```python
from build123d import *

# Parameters (mm, degrees)
F1_DEPTH = 30
F2_R     = 10
F3_R     = 10
F4_R     = 10
F5_R     = 10
F6_W     = 10
F6_H     = 10
F6_R     = 0.75
F7_DEPTH = 2


with BuildPart() as f1:
    # F0 (on Front) → F1 (new body)
    with BuildSketch(Plane.XZ):
        Polygon((40, 0), (0, 0), (-40, 0), (-48.660254, 5), (-51.324189, 0.768753), (-41.332416, -5), (41.336155, -5), (51.275389, 0.73842), (48.660254, 5), align=None)
    extrude(amount=F1_DEPTH)

    # F2
    f2_edges = [f1.edges().sort_by_distance(p)[0] for p in [
        (49.967822, -30, 2.86921),
    ]]
    fillet(f2_edges, radius=F2_R)

    # F3
    f3_edges = [f1.edges().sort_by_distance(p)[0] for p in [
        (49.967822, 0, 2.86921),
    ]]
    fillet(f3_edges, radius=F3_R)

    # F4
    f4_edges = [f1.edges().sort_by_distance(p)[0] for p in [
        (-49.992221, 0, 2.884377),
    ]]
    fillet(f4_edges, radius=F4_R)

    # F5
    f5_edges = [f1.edges().sort_by_distance(p)[0] for p in [
        (-49.992221, -30, 2.884377),
    ]]
    fillet(f5_edges, radius=F5_R)

    # F6 (on face) → F7 (join)
    with BuildSketch(Plane(origin=(0, 0, -5), x_dir=(1, 0, 0), z_dir=(0, 0, -1))):
        with Locations((31.332416, 15)):
            Rectangle(F6_W, F6_H)
        with Locations((28.082416, 11.75)):
            Circle(F6_R, mode=Mode.SUBTRACT)
        with Locations((34.582416, 11.75)):
            Circle(F6_R, mode=Mode.SUBTRACT)
        with Locations((28.082416, 18.25)):
            Circle(F6_R, mode=Mode.SUBTRACT)
        with Locations((34.582416, 18.25)):
            Circle(F6_R, mode=Mode.SUBTRACT)
        with Locations((-31.332416, 15)):
            Rectangle(F6_W, F6_H)
        with Locations((-34.582416, 11.75)):
            Circle(F6_R, mode=Mode.SUBTRACT)
        with Locations((-28.082416, 11.75)):
            Circle(F6_R, mode=Mode.SUBTRACT)
        with Locations((-34.582416, 18.25)):
            Circle(F6_R, mode=Mode.SUBTRACT)
        with Locations((-28.082416, 18.25)):
            Circle(F6_R, mode=Mode.SUBTRACT)
    extrude(amount=F7_DEPTH)


solid = f1.part
```
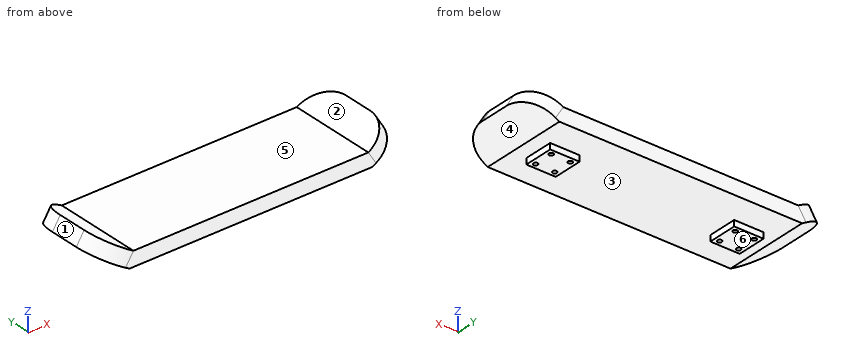
Input: part model. Units: mm. Frame: model coordinates. Face numbers are marked on the shaded views. A direction names the side the tool comes from. Coordinates: 2 decimals unless noted, no trailing zeros. Write each loop counter-clockwise with the first axis right and the second up, starting at its lowest first coordinate (ties: lowest second). Pieces come first, ordered by that corner, then holes. Notation, with made-up numbers: (8, 57.5) - (29, 57.5) arc R23 cw to (29, 71.5) - close; hole circle Ø1 at (70, 41.25). An arc over 180 degrees is marked (long way). Put each result on its own line as item: value. Start each with the question number.
1) Reachability of the marked faces 5 and 6 from +Z, -Z, +X, -X, +Y, -Y: full face, straight path, thin tool, end or side. Return the list, or none.
2) Cut plane C-C (y = -21.25). Return the cut outline in (x, z), plus the area to 3 significant figures.
3) Contact query for flat-ended pins moving along their axis: pin 1 (2 mm diameter, centred on x = 32.5, z = -5.5, fed in from +Y); pin 2 (15 mm diameter, centred on x = 7, y = -19.5, fed in from +Z); pin 3 (1.6 mm diameter, centred on y = -16.5, z = -6.5, fed in from +X); pin 4 (2 mm diameter, centred on y = -8, z = -2.5, fed in from -X). Output: stop coordinate, or through.
4) Cut plane B-B (x = 0). Return the cut outline in (y, z), plus the area to 3 significant figures.
5) Ray query, L1, parallel to X at y = -11.75, z = -5.5; L2, parallel to Z at x = 24, y = -8.25; L3, parallel to X at y = -10.25, z = 1. Return the intervals inside material, ascending.
6) Cut plane A-A (y = -5.75). Return the cut outline in (x, z).
7) Mould query, pull axis X, two halves, no side actions, for the marked faces 1, 2, 3 and 4. Classes: pulls with the +X half, pulls with the -X half, needs draft (parallel to the pull), parting line crosses it, or undercut.
Resolved:
1. face 5: +Z, +Y, -Y
1. face 6: -Z, +X, -X, +Y, -Y
2. outline: (-51.26, 0.73) - (-41.33, -5) - (41.34, -5) - (51.21, 0.7) - (48.59, 4.96) - (40, 0) - (-40, 0) - (-48.59, 4.96) - close
2. area: 513 mm2
3. pin 1: stops at y = 0
3. pin 2: stops at z = 0
3. pin 3: stops at x = 36.33
3. pin 4: stops at x = -47.39
4. outline: (-30, -5) - (0, -5) - (0, 0) - (-30, 0) - close
4. area: 150 mm2
5. L1: x = -36.33 to -35.33, -33.83 to -28.83, -27.33 to -26.33, 26.33 to 27.33, 28.83 to 33.83, 35.33 to 36.33
5. L2: z = -5 to 0
5. L3: x = -51.18 to -41.73, 41.73 to 51.11
6. outline: (-50.5, 0.29) - (-41.33, -5) - (41.34, -5) - (50.45, 0.26) - (47.84, 4.53) - (40, 0) - (-40, 0) - (-47.84, 4.53) - close
7. face 1: pulls with the -X half
7. face 2: undercut
7. face 3: undercut
7. face 4: pulls with the +X half
